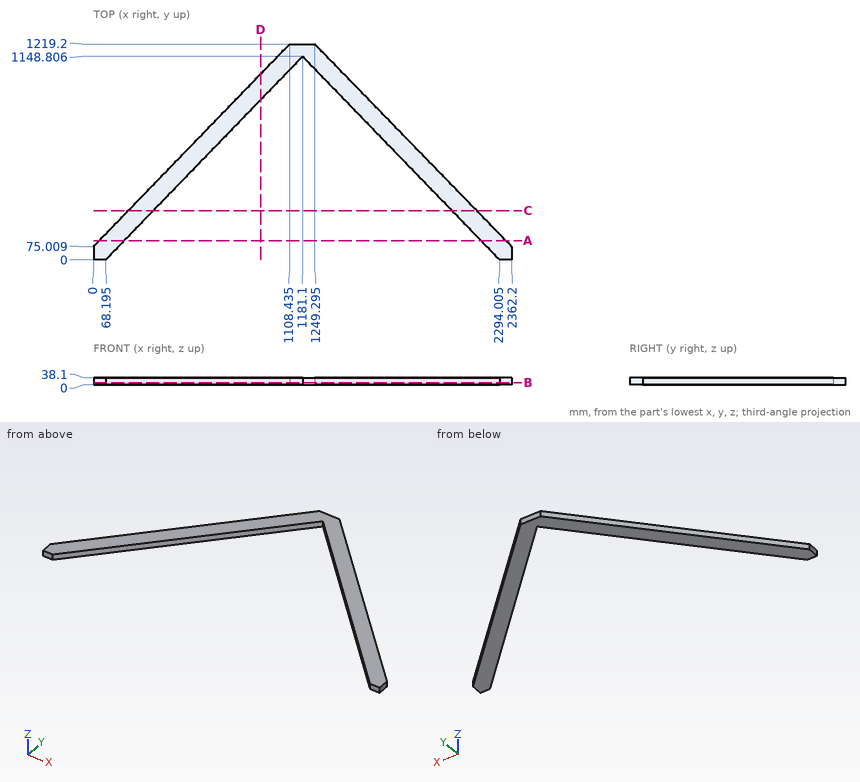
Verification items for this drawing (mm, ordinates from the low corner). Round coordinates to 2 decimals unless told otherwise and drop trailing zeros. Write each loop counter-clockwise with the first axis right and the second up, starting at its lowest first coordinate (ties: lowest second). Pieces come first, ordered by that corner, then holes. Notation, with made-up numbers: (-30, 19.5) - (-8, 19.5) arc R33 cw to (-8, 50.5) - close; hole circle Ø3 at (-7.5, -29). An arc over 180 degrees is marked (long way). One line per item, written item: value.
1. Depth check by flat-ended pin: pin 1 Ø3 at (x, z) = (1803, 12) entering from +Y; pin 2 Ø6 at (y, z) = (792, 20.5) entering from +X; pin 3 Ø1.5 at (x, z) = (287.5, 9) entering from +Y. Enter the tip coordinate at first touch or a pass-through.
The answers:
pin 1: stops at y = 651.47
pin 2: stops at x = 1667.73
pin 3: stops at y = 372.56
2. Cross-section at C-C on y = 278.5. Record the boundary of the cut face in (x, z), and give its area (3 significant figures).
The answers:
outline: (197.13, 0) - (337.99, 0) - (337.99, 38.1) - (197.13, 38.1) - close; (2024.21, 0) - (2164.27, 0) - (2164.27, 38.1) - (2024.21, 38.1) - close
area: 10,700 mm^2
3. Scan lines: L1, parallel to X at y = 1136.5, z = 22.5 (1 decimal); L2, parallel to X at y = 708.5, z = 12.5 (1 decimal); L3, parallel to Y at x = 370, z = 25 (1 decimal). Record each from-to range of solid material in increasing order.
The answers:
L1: x = 1028.3 to 1169.2, 1193 to 1329.7
L2: x = 613.7 to 754.6, 1607.6 to 1746
L3: y = 311.5 to 456.9
4. Cross-section at B-B on z = 11. Record the boundary of the cut face in (x, y) (1 decimal), and give its area (3 significant figures).
The answers:
outline: (0, 0) - (68.2, 0) - (1181.1, 1148.8) - (2294, 0) - (2362.2, 0) - (2362.2, 75) - (1249.3, 1219.2) - (1108.4, 1219.2) - (0, 75) - close
area: 331,000 mm^2
5. Cross-section at A-A on y = 108. Record the boundary of the cut face in (x, z).
The answers:
outline: (31.96, 0) - (172.82, 0) - (172.82, 38.1) - (31.96, 38.1) - close; (2189.38, 0) - (2330.11, 0) - (2330.11, 38.1) - (2189.38, 38.1) - close
6. Cross-section at D-D on x = 944. Record the boundary of the cut face in (y, z).
The answers:
outline: (904.06, 0) - (1049.46, 0) - (1049.46, 38.1) - (904.06, 38.1) - close
